```python
from build123d import *

# Parameters (mm, degrees)
SKETCH1_R           = 6.7
SKETCH1_R_2         = 1.586
BOSS_EXTRUDE1_DEPTH = 7.4
SKETCH2_R           = 3.5
SKETCH2_R_2         = 1.586
BOSS_EXTRUDE2_DEPTH = 7.54
SKETCH3_R           = 1.25
CUT_EXTRUDE1_DEPTH  = 10


with BuildPart() as part:
    # Sketch1 → Boss-Extrude1 (new body)
    with BuildSketch(Plane(origin=(0, 0, 0), x_dir=(1, 0, 0), z_dir=(0, 1, 0))):
        Circle(SKETCH1_R)
        Circle(SKETCH1_R_2, mode=Mode.SUBTRACT)
    extrude(amount=BOSS_EXTRUDE1_DEPTH)

    # Sketch2 → Boss-Extrude2 (add)
    with BuildSketch(Plane.XZ):
        Circle(SKETCH2_R)
        Circle(SKETCH2_R_2, mode=Mode.SUBTRACT)
    extrude(amount=BOSS_EXTRUDE2_DEPTH)

    # Sketch3 → Cut-Extrude1 (cut)
    with BuildSketch(Plane(origin=(0, 0, 0), x_dir=(0, 0, -1), z_dir=(1, 0, 0))):
        with Locations((0, -3.77)):
            Circle(SKETCH3_R)
    extrude(amount=-CUT_EXTRUDE1_DEPTH, mode=Mode.SUBTRACT)


solid = part.part
```
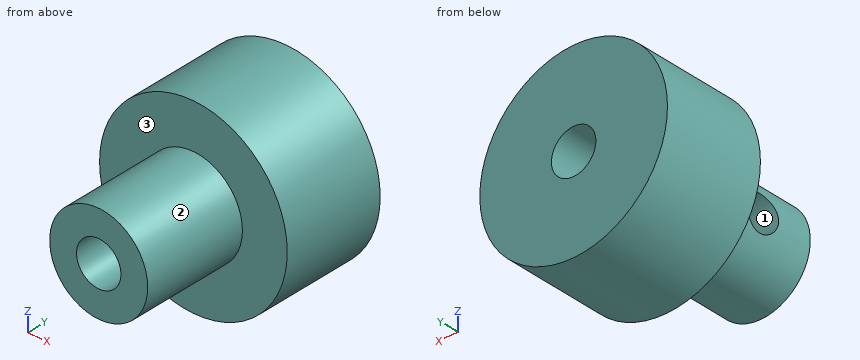
Work out the finished part from the listing and answer in its coordinate system (mm). Face numbers are marked on the shaded views. Coordinates: 2 decimals unless noted, no trailing zeros. Loops run counter-clockwise (first coordinate to the right, second up) from the corner with the lowest first, then second, coordinate; pieces in that order, holes last. Notation, with made-up numbers: M -23,-8.5 L -1,-8.5 A29 cw -1,24.5 Z; hole C 41,-33.75 d9. An arc over 180 degrees is marked long. Use CSV: the item, a comma, the result in double quotes. Start each with the question number.
(1) Find section A-A, the plane x = 0. Give the vertices of the cut face in (y, z).
(2) For a pull along Z with two mould halves and no side action, classify the marked faces 1, 2 and 3 as +Z half, -Z half, draft (parallel to the pull), parting line (faces both ways), or undercut.
(3) Find section B-B, the plane x = -2.25. Give the vertices of the cut face in (y, z), then the cut area to 3 significant figures.
(4) Given pin 1 Ø8 at (x, y) = (-5.5, 4.5) entering from +Z; pin 2 Ø5 at (y, z) = (0.5, 1.5) entering from -X; pin 3 Ø3 at (x, y) = (-4, -5.5) entering from +Z; pin 4 Ø3 at (y, z) = (-3.77, 0) entering from -X, each flat-ended and moving along its own axis, determine where each tip first touches the part or whether it passes through.
(5) Find section D-D, the plane z = 2.5. Give the vertices of the cut face in (x, y), then the cut area to 3 significant figures.
(6) Find section C-C, the plane y = -5.75. Give the vertices of the cut face in (x, z), then the cut area to 3 significant figures.
(7) Consider line 1 (X direction, y = 3.5, z = 0); line 2 (X direction, y = -3, z = 0); line 3 (Y direction, x = 0, z = -6). Determine where each line is inside the solid, lowest interval first.
Recorded:
1,outline,"M -7.54,-3.5 L 0,-3.5 L 0,-6.7 L 7.4,-6.7 L 7.4,-1.59 L -7.54,-1.59 Z; M -7.54,1.59 L 7.4,1.59 L 7.4,6.7 L 0,6.7 L 0,3.5 L -7.54,3.5 Z"
2,face 1,"undercut"
2,face 2,"parting line"
2,face 3,"draft"
3,outline,"M -7.54,-2.68 L 0,-2.68 L 0,-6.31 L 7.4,-6.31 L 7.4,6.31 L 0,6.31 L 0,2.68 L -7.54,2.68 Z; hole C -3.77,0 d2.5"
3,area,"129 mm^2"
4,pin 1,"stops at z = 6.53"
4,pin 2,"stops at x = -6.7"
4,pin 3,"stops at z = 2.45"
4,pin 4,"stops at x = -3.5"
5,outline,"M -6.22,0 L -2.45,0 L -2.45,-7.54 L 2.45,-7.54 L 2.45,0 L 6.22,0 L 6.22,7.4 L -6.22,7.4 Z"
5,area,"129 mm^2"
6,outline,"C 0,0 d7; hole C 0,0 d3.17"
6,area,"30.6 mm^2"
7,line 1,"x = -6.7 to -1.59, 1.59 to 6.7"
7,line 2,"x = 1.59 to 3.5"
7,line 3,"y = 0 to 7.4"
